Source: three-view drawing plus pictorial views. Frame: mm from the lowest corner of the part. A direction names the side the tool comes from. Give positions to 0.01 mm unless a question says otherwise; leave off trailing zeros. Write each loop counter-clockwise with the first axis right and the second up, starting at its lowest first coordinate (ties: lowest second). Pieces come first, ordered by that corner, then holes. Notation, with made-up numbers: (47.5, -29) -> (86.5, -29) arc R18 ccw to (86.5, -20) -> close; hole circle Ø9 at (55.5, -29). An arc over 180 degrees is marked (long way). Write item = value, one per line.
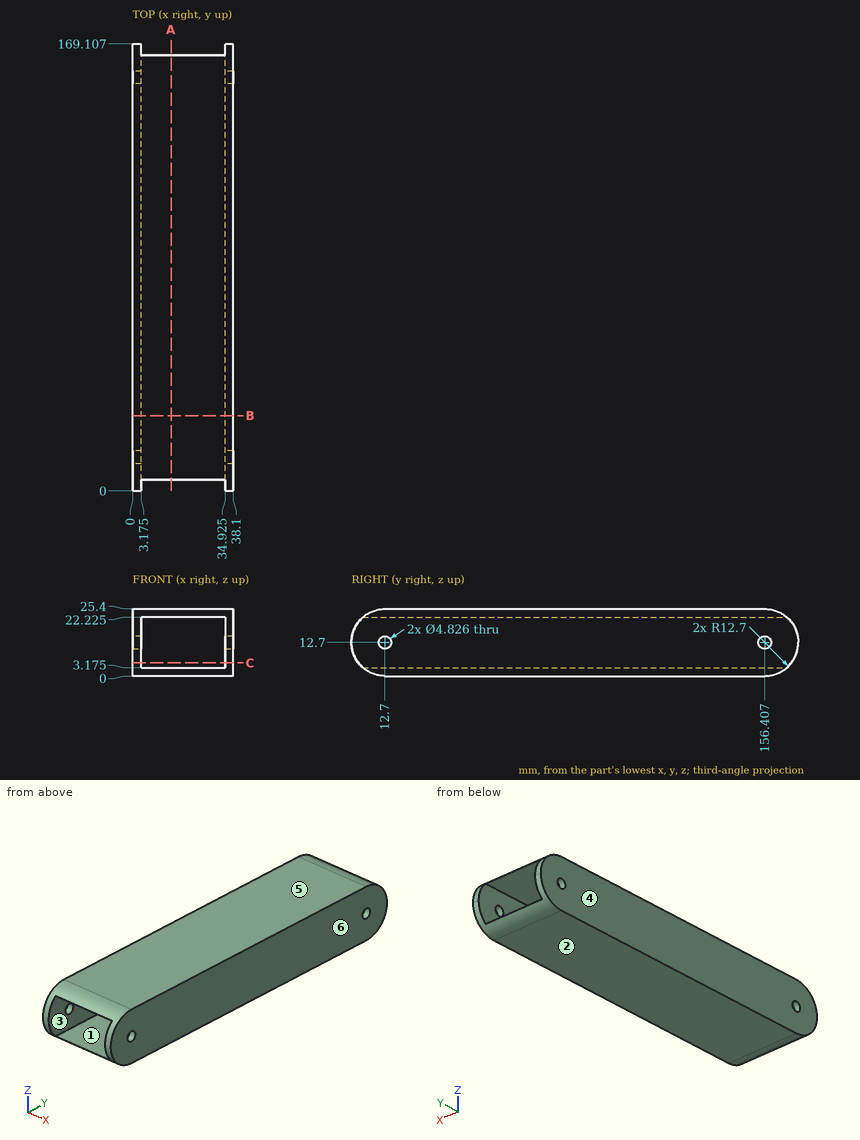
1) Access query for the marked faces 1 and 2. Directions: +Z, -Z, +X, -X, +Y, -Y. A direction counts if a zero-diameter tool reaches every point of the face in a straight line with its end or side. Return the directions, or none.
Computed:
face_1 = +Y, -Y
face_2 = -Z, +X, -X, +Y, -Y
2) Cut plane C-C (z = 5). Return the cut outline in (x, y) (1 decimal).
Computed:
outline = (0, 2.6) -> (3.2, 2.6) -> (3.2, 166.5) -> (0, 166.5) -> close; (34.9, 2.6) -> (38.1, 2.6) -> (38.1, 166.5) -> (34.9, 166.5) -> close
3) Contact query for flat-ended pins moving along their axis: pin 1 (4 mm diameter, centred on y = 12.7, z = 12.7, fed in from +X); pin 2 (7.5 mm diameter, centred on y = 156.41, z = 12.7, fed in from +X). Output: stop coordinate, or through.
Computed:
pin_1 = through
pin_2 = 38.1
4) Cut plane B-B (y = 28.5). Return the cut outline in (x, z) (1 decimal).
Computed:
outline = (0, 0) -> (38.1, 0) -> (38.1, 25.4) -> (0, 25.4) -> close; hole (3.2, 3.2) -> (34.9, 3.2) -> (34.9, 22.2) -> (3.2, 22.2) -> close
5) Material intervals for L1, parallel to Z at x = 24.5, y = 65 (1 decimal); L2, parallel to X at y = 46, z = 18.75 (1 decimal); L3, parallel to Y at x = 1.55, z = 12.7, sorted ascending.
Computed:
L1 = 0 to 3.2, 22.2 to 25.4
L2 = 0 to 3.2, 34.9 to 38.1
L3 = 0 to 10.29, 15.11 to 153.99, 158.82 to 169.11
6) Draft query along X for the marked faces 3, 4, 5 and 6. Return one class per face: pulls with the +X half, pulls with the -X half, needs draft (parallel to the pull), parting line crosses it, or undercut.
Computed:
face_3 = undercut
face_4 = pulls with the -X half
face_5 = needs draft
face_6 = pulls with the +X half
7) Cut plane A-A (x = 14.5). Return the cut outline in (y, z) (1 decimal).
Computed:
outline = (4.3, 3.2) arc R12.7 ccw to (12.7, 0) -> (156.4, 0) arc R12.7 ccw to (164.8, 3.2) -> close; (4.3, 22.2) -> (164.8, 22.2) arc R12.7 ccw to (156.4, 25.4) -> (12.7, 25.4) arc R12.7 ccw to start
